from build123d import *

# Parameters (mm, degrees)
CYLINDER010_R     = 1
CYLINDER010_DEPTH = 10
BOX017_W          = 13
BOX017_H          = 5
BOX017_DEPTH      = 6
CHAMFER001_SIZE   = 4.5


with BuildPart() as cilindro010:
    # Cylinder010 → Cylinder010 (new body)
    with BuildSketch(Plane(origin=(15, 4.5, 113), x_dir=(1, 0, 0), z_dir=(0, 0, 1))):
        Circle(CYLINDER010_R)
    extrude(amount=CYLINDER010_DEPTH)


with BuildPart() as sim:
    # Box017 → Box017 (new body)
    with BuildSketch(Plane(origin=(4, 2, 118), x_dir=(1, 0, 0), z_dir=(0, 0, 1))):
        with Locations((6.5, 2.5)):
            Rectangle(BOX017_W, BOX017_H)
    extrude(amount=BOX017_DEPTH)

    # Chamfer001
    chamfer001_edges = [sim.edges().sort_by_distance(p)[0] for p in [
        (10.5, 7, 124),
    ]]
    chamfer(chamfer001_edges, length=CHAMFER001_SIZE)

    # Cut030: cut Cilindro010
    add(cilindro010.part, mode=Mode.SUBTRACT)


solid = sim.part
Source: CAD feature listing. Evaluate the final solid. Frame: model axes, mm. Coordinates: 2 decimals unless noted, no trailing zeros. Order: outer loops, then holes, each group sorted by start corner. A loop starts at its lowest first (then second) coordinate and runs counter-clockwise, first axis right, second up. Notation, with made-up numbers: M -1,12 L 44,12 A23 cw 44,33 Z; hole C -3,-26 d5. An arc over 180 degrees is marked long. Write each question's results on one line, items separated by ' | '. Start each with the question number.
Item 1: Cut plane C-C (z = 120.5). Return loops of the section in (x, y).
Item 2: Cut plane A-A (y = 4.5). Return loops of the section in (x, z), and give its area (3 significant figures).
Item 3: Cut plane B-B (x = 15). Return loops of the section in (y, z).
Item 4: First-contact query: pin 1 Ø1.5 at (x, z) = (12, 123) entering from +Y; pin 2 Ø3 at (x, y) = (15, 4.5) entering from +Z; pin 3 Ø3 at (x, y) = (9.5, 6.5) entering from +Z. Flat tips, straight axial feed; report the tip coordinate or a pass-through.
Item 5: Cut plane D-D (x = 5.5). Return loops of the section in (y, z).
Item 6: Line query: probe 1 along X at (y, z) = (4.5, 119.4); probe 2 along Y at (x, z) = (15, 119.3); probe 3 along Y at (x, z) = (15, 120.4). Output: solid intervals per line, ascending.
Checked values:
1) outline: M 4,2 L 17,2 L 17,6 L 4,6 Z; hole C 15,4.5 d2
2) outline: M 4,118 L 14,118 L 14,122 L 4,122 Z; M 16,118 L 17,118 L 17,122 L 16,122 Z | area: 44.0 mm2
3) outline: M 2,118 L 3.5,118 L 3.5,123 L 2.5,124 L 2,124 Z; M 5.5,118 L 7,118 L 7,119.5 L 5.5,121 Z
4) pin 1: stops at y = 4.25 | pin 2: stops at z = 123.5 | pin 3: stops at z = 121.5
5) outline: M 2,118 L 7,118 L 7,119.5 L 2.5,124 L 2,124 Z
6) probe 1: x = 4 to 14, 16 to 17 | probe 2: y = 2 to 3.5, 5.5 to 7 | probe 3: y = 2 to 3.5, 5.5 to 6.1
